```python
from build123d import *

# Parameters (mm, degrees)
BOSS_EXTRUDE1_DEPTH = 20
FILLET1_R           = 30
FILLET2_R           = 35
SKETCH2_W           = 5
SKETCH2_H           = 20
BOSS_EXTRUDE2_DEPTH = 15
SKETCH3_R           = 1.4
CUT_EXTRUDE1_DEPTH  = 45


with BuildPart() as part:
    # Sketch1 → Boss-Extrude1 (new body)
    with BuildSketch(Plane.XY):
        Polygon((11.448507825, 54.464802922), (6.448507825, 54.464802922), (6.448507825, 44.464802922), (-8.551492175, 44.464802922), (-13.551492175, 44.464802922), (-13.551492175, 39.464802922), (-13.551492175, -50.535197078), (-13.551492175, -55.535197078), (-8.551492175, -55.535197078), (46.448507825, -55.535197078), (46.448507825, -50.535197078), (-8.551492175, -50.535197078), (-8.551492175, 39.464802922), (6.448507825, 39.464802922), (36.448507825, 39.464802922), (36.448507825, 54.464802922), (31.448507825, 54.464802922), (31.448507825, 44.464802922), (11.448507825, 44.464802922), align=None)
    extrude(amount=BOSS_EXTRUDE1_DEPTH)

    # Fillet1
    fillet1_edges = [part.edges().sort_by_distance(p)[0] for p in [
        (-8.551492175, 39.464802922, 10),
        (-8.551492175, -50.535197078, 10),
    ]]
    fillet(fillet1_edges, radius=FILLET1_R)

    # Fillet2
    # the kernel refuses this fillet: 35 mm, written as the material it takes off along each edge
    with BuildSketch(Plane(origin=(-13.551492175, -55.535197078, -87.5), x_dir=(1, 0, 0), z_dir=(0, 0, 1))) as fillet2_piece_1:
        with BuildLine():
            CenterArc((FILLET2_R, FILLET2_R), FILLET2_R, 180, 90)
            Line((0, FILLET2_R), (-FILLET2_R * 0.02, FILLET2_R))
            Line((-FILLET2_R * 0.02, FILLET2_R), (-FILLET2_R * 0.02, -FILLET2_R * 0.02))
            Line((-FILLET2_R * 0.02, -FILLET2_R * 0.02), (FILLET2_R, -FILLET2_R * 0.02))
            Line((FILLET2_R, -FILLET2_R * 0.02), (FILLET2_R, 0))
        make_face()
    extrude(amount=195, mode=Mode.SUBTRACT)
    with BuildSketch(Plane(origin=(-13.551492175, 44.464802922, -79.056941504), x_dir=(0, -1, 0), z_dir=(0, 0, 1))) as fillet2_piece_2:
        with BuildLine():
            CenterArc((31.622776602, 35), FILLET2_R, 205.376933525, 64.623066475)
            Line((0, 20), (-0.632455532, 19.7))
            ThreePointArc((-0.632455532, 19.7), (-0.7, 10), (-0.7, 0))
            Line((-0.7, 0), (0, -0.7))
            Line((0, -0.7), (31.622776602, -0.7))
            Line((31.622776602, -0.7), (31.622776602, 0))
        make_face()
    extrude(amount=178.113883008, mode=Mode.SUBTRACT)

    # Sketch2 → Boss-Extrude2 (add)
    with BuildSketch(Plane(origin=(0, 54.464802922, 0), x_dir=(1, 0, 0), z_dir=(0, 1, 0))):
        with Locations((8.948507825, -10)):
            Rectangle(SKETCH2_W, SKETCH2_H)
        with Locations((33.948507825, -10)):
            Rectangle(SKETCH2_W, SKETCH2_H)
    extrude(amount=BOSS_EXTRUDE2_DEPTH)

    # Sketch3 → Cut-Extrude1 (cut)
    with BuildSketch(Plane(origin=(36.448507825, 0, 0), x_dir=(0, 0, -1), z_dir=(1, 0, 0))):
        with Locations(Location((-10, 66.264802922, 0), (0, 0, 90))):
            Circle(SKETCH3_R)
    extrude(amount=-CUT_EXTRUDE1_DEPTH, mode=Mode.SUBTRACT)


solid = part.part
```
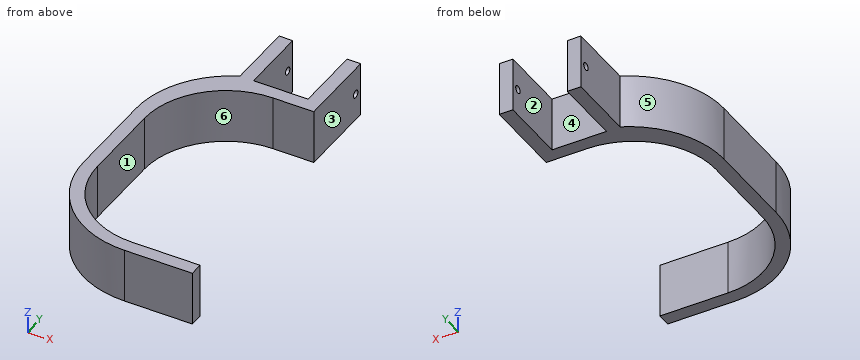
Verification items for the finished model (mm, model axes). Face numbers are marked on the shaded views. A direction names the side the tool comes from. Give positions to 0.01 mm unless a question says otherwise; leave off trailing zeros. Order: outer loops, then holes, each group sorted by start corner. A loop starts at its lowest first (then second) coordinate and runs counter-clockwise, first axis right, second up. Notation, with made-up numbers: (-27.5, 82) -> (-18.5, 82) arc R23 cw to (-18.5, 113) -> close; hole circle Ø11 at (32.25, 81.25). An arc over 180 degrees is marked (long way). Use a Markdown table: item, result.
1) Section check D-D, the plane y = -3. Record the boundary of the cut face in (x, z), then the cut area to 3 significant figures.
Results:
| item | result |
|---|---|
| outline | (-13.55, 0) -> (-8.55, 0) -> (-8.55, 20) -> (-13.55, 20) -> close |
| area | 100 mm² |
2) Section check A-A, the plane z = 10. Record the boundary of the cut face in (x, y), then the cut area to 3 significant figures.
Results:
| item | result |
|---|---|
| outline | (-13.55, -20.54) arc R35 ccw to (21.45, -55.54) -> (46.45, -55.54) -> (46.45, -50.54) -> (21.45, -50.54) arc R30 cw to (-8.55, -20.54) -> (-8.55, 9.46) arc R30 cw to (21.45, 39.46) -> (36.45, 39.46) -> (36.45, 64.86) -> (31.45, 64.86) -> (31.45, 44.46) -> (11.45, 44.46) -> (11.45, 64.86) -> (6.45, 64.86) -> (6.45, 44.46) arc R35 ccw to (-13.55, 12.84) -> close; (6.45, 67.66) -> (11.45, 67.66) -> (11.45, 69.46) -> (6.45, 69.46) -> close; (31.45, 67.66) -> (36.45, 67.66) -> (36.45, 69.46) -> (31.45, 69.46) -> close |
| area | 1,170 mm² |
3) Depth check by flat-ended pin: pin 1 Ø3.5 at (y, z) = (66.26, 10) entering from +X; pin 2 Ø3 at (y, z) = (-26.5, 16.5) entering from +X; pin 3 Ø2 at (x, z) = (-1.5, 13.5) entering from +Y; pin 4 Ø1.7 at (y, z) = (66.26, 10) entering from -X. Enter the tip coordinate at first touch or a pass-through.
Results:
| item | result |
|---|---|
| pin 1 | x = 36.45 |
| pin 2 | x = -7.61 |
| pin 3 | y = 40.1 |
| pin 4 | through |
4) Tool access check on the marked faces 1, 2 and 3. Record the directions out of +Z, -Z, +X, -X, +Y, -Y that give a thin tool (end or side, any length) a straight path to the whole face; none if there is none.
Results:
| item | result |
|---|---|
| face 1 | +Z, -Z, +X |
| face 2 | +Z, -Z, +Y |
| face 3 | +Z, -Z, +X, +Y |
5) Section check C-C, the plane x = 2.5. Record the boundary of the cut face in (y, z), then the cut area to 3 significant figures.
Results:
| item | result |
|---|---|
| outline | (-49.96, 0) -> (-43.79, 0) -> (-43.79, 20) -> (-49.96, 20) -> close; (32.72, 0) -> (42.27, 0) -> (42.27, 20) -> (32.72, 20) -> close |
| area | 314 mm² |
6) Material ranges on probe 1 along X at (y, z) = (62, 2.5); probe 2 along Y at (x, z) = (27.5, 14); probe 3 along Y at (x, z) = (31.5, 16.75), recorded low to high.
Results:
| item | result |
|---|---|
| probe 1 | 6.45 to 11.45, 31.45 to 36.45 |
| probe 2 | -55.54 to -50.54, 39.46 to 44.46 |
| probe 3 | -55.54 to -50.54, 39.46 to 69.46 |
7) Mould release check, pull along X, two halves, no side actions. Record for the marked faces 4, 5 and 6: pulls with the +X half, pulls with the -X half, needs draft (parallel to the pull), parting line crosses it, or undercut.
Results:
| item | result |
|---|---|
| face 4 | undercut |
| face 5 | pulls with the -X half |
| face 6 | pulls with the +X half |
8) Section check B-B, the plane x = 9. Record the boundary of the cut face in (y, z).
Results:
| item | result |
|---|---|
| outline | (-53.25, 0) -> (-47.83, 0) -> (-47.83, 20) -> (-53.25, 20) -> close; (36.76, 0) -> (69.46, 0) -> (69.46, 20) -> (36.76, 20) -> close; hole circle Ø2.8 at (66.26, 10) |
